from build123d import *

# Parameters (mm, degrees)
F0_R     = 12.5
F1_DEPTH = 3


with BuildPart() as f1:
    # F0 (on Top) → F1 (new body)
    with BuildSketch(Plane.XY):
        with BuildLine():
            Line((15, -9.0138781887), (15, 9.0138781887))
            ThreePointArc((15, 9.0138781887), (-17.5, 0), (15, -9.0138781887))
        make_face()
        Circle(F0_R, mode=Mode.SUBTRACT)
        with BuildLine():
            ThreePointArc((15, -9.0138781887), (16.863421954, -4.6770717335), (17.5, 0))
            ThreePointArc((17.5, 0), (16.863421954, 4.6770717335), (15, 9.0138781887))
            Line((15, 9.0138781887), (15, -9.0138781887))
        make_face()
        with BuildLine():
            ThreePointArc((15, 9.0138781887), (16.863421954, 4.6770717335), (17.5, 0))
            ThreePointArc((17.5, 0), (16.863421954, -4.6770717335), (15, -9.0138781887))
            Line((15, -9.0138781887), (15, -17.5))
            Line((15, -17.5), (20, -17.5))
            Line((20, -17.5), (20, 17.5))
            Line((20, 17.5), (15, 17.5))
            Line((15, 17.5), (15, 9.0138781887))
        make_face()
    extrude(amount=F1_DEPTH)


solid = f1.part
Verification items for the finished model (mm, model axes). A direction names the side the tool comes from. Coordinates: 2 decimals unless noted, no trailing zeros. Loops run counter-clockwise (first coordinate to the right, second up) from the corner with the lowest first, then second, coordinate; pieces in that order, holes last. Notation, with made-up numbers: M 56,-4 L 74,-4 A19 cw 74,26 Z; hole C -4.75,79 d8. An arc over 180 degrees is marked long. One line per item, written item: value.
1. Section check C-C on y = -11.5. Record the cut outline in (x, z), plus the area to 3 significant figures.
Answers follow:
outline: M -13.19,0 L -4.9,0 L -4.9,3 L -13.19,3 Z; M 4.9,0 L 13.19,0 L 13.19,3 L 4.9,3 Z; M 15,0 L 20,0 L 20,3 L 15,3 Z
area: 64.8 mm^2
2. Section check A-A on x = 0. Record the cut outline in (y, z), plus the area to 3 significant figures.
Answers follow:
outline: M -17.5,0 L -12.5,0 L -12.5,3 L -17.5,3 Z; M 12.5,0 L 17.5,0 L 17.5,3 L 12.5,3 Z
area: 30.0 mm^2
3. Gauge pin test, flat ends, axial feed: P1, Ø1.5, axis at x = -1, z = 1, coming from the +Y side; P2, Ø0.9, axis at y = -13, z = 1.5, coming from the -X side; P3, Ø1, axis at x = -1, z = 2, coming from the -Y side. Record the tip position at first contact, or that the pin passes through.
Answers follow:
P1: y = 17.5
P2: x = -12.2
P3: y = -17.49
4. Mould release check, pull along X, two halves, no side actions. Record for faces 4 (the flat face through (13, 0, 0)), 5 (the flat face through (20, 0, 1)), 6 (the cylindrical face through (11.923, 3.755, 1.479)): pulls with the +X half, pulls with the -X half, needs draft (parallel to the pull), parting line crosses it, or undercut.
Answers follow:
face 4: needs draft
face 5: pulls with the +X half
face 6: undercut
5. Section check B-B on y = 0. Record the cut outline in (x, z), plus the area to 3 significant figures.
Answers follow:
outline: M -17.5,0 L -12.5,0 L -12.5,3 L -17.5,3 Z; M 12.5,0 L 20,0 L 20,3 L 12.5,3 Z
area: 37.5 mm^2
6. Set-up check for faces 1 (the flat face through (15, 13, 1)), 2 (the flat face through (15, -13, 1)), 3 (the flat face through (13, 0, 3)): record each of +Z, -Z, +X, -X, +Y, -Y from which the full face is reachable in a straight line by a thin tool's end or side.
Answers follow:
face 1: +Z, -Z, +Y
face 2: +Z, -Z, -Y
face 3: +Z, +X, -X, +Y, -Y
7. Material ranges on line 1 along Y through (x, z) = (0, 0.75); line 2 along X through (y, z) = (10, 1.2); line 3 along Y through (x, z) = (4.5, 2.5), recorded low to high. Write a range as from..to.
Answers follow:
line 1: -17.5..-12.5, 12.5..17.5
line 2: -14.36..-7.5, 7.5..14.36, 15..20
line 3: -16.91..-11.66, 11.66..16.91
8. Section check D-D on z = 1.4. Record the cut outline in (x, y), plus the area to 3 significant figures.
Answers follow:
outline: M 15,-17.5 L 20,-17.5 L 20,17.5 L 15,17.5 L 15,9.01 A17.5 ccw long 15,-9.01 Z; hole C 0,0 d25
area: 616 mm^2
